Autodesk Inventor part; units mm, degrees
ref_plane "YZ Plane" through (0, 0, 0) normal (1, 0, 0) x (0, 1, 0)
ref_plane "XZ Plane" through (0, 0, 0) normal (0, 1, 0) x (-1, 0, 0)
ref_plane "XY Plane" through (0, 0, 0) normal (0, 0, 1) x (1, 0, 0)
sketch "Schizzo1" plane through (0, 0, 0) normal (0, 1, 0) x (-1, 0, 0)
  line L0 (-15, 6) -> (-15, 10.5)
  line L1 (-15, 10.5) -> (-11.5, 10.5)
  line L2 (-11.5, 10.5) -> (-11.5, 10)
  line L3 (-11.5, 10) -> (-10.2, 10)
  line L4 (-10.2, 10) -> (-10.2, 10.5)
  line L5 (-10.2, 10.5) -> (0, 10.5)
  line L6 (0, 10.5) -> (0, 6)
  line L7 (0, 6) -> (-15, 6)
  line L8 (0, 0) -> (5.7518, 0)
  dimension "d0" = 12
  dimension "d2" = 21
  dimension "d3" = 15
  dimension "d4" = 11.5
  dimension "d5" = 1.3
  dimension "d6" = 20
revolve "Rivoluzione1" add sketch "Schizzo1" angle 360 about axis through (0, 0, 0) along (-1, 0, 0)
fillet "Raccordo1" radius 0.2 1 edges at (15, 0, -10.5)
sketch "Schizzo2" plane through (15, 0, 0) normal (1, 0, 0) x (0, 0, -1)
  circle A0 centre (0, 0) radius 10.3
  circle A1 centre (0, 0) radius 9
  dimension "d13" = 18
extrude "Estrusione2" cut sketch "Schizzo2" against normal blind 1 contours A1
mirror "Specchio1" about plane through (0, 0, 8.25) normal (-1, 0, 0)
properties part number "LM10UU"
Work out the finished part from the listing and answer in its coordinate system (mm). A direction names the side the tool comes from. Coordinates: 2 decimals unless noted, no trailing zeros. Order: outer loops, then holes, each group sorted by start corner. A loop starts at its lowest first (then second) coordinate and runs counter-clockwise, first axis right, second up. Notation, with made-up numbers: M -18,67 L 20,67 A26 ccw 20,85 Z; hole C 70,-2 d11. An arc over 180 degrees is marked long. Use CSV: the item, a comma, the result in double quotes.
1) Section A-A on x = 6.5 is taken. Write down the section's boundary in (y, z), plus the area to 3 significant figures.
Worked out:
outline,"C 0,0 d21; hole C 0,0 d12"
area,"233 mm^2"
2) For faces 1 (the face through (-14, -6, 2)), 2 (the face through (10.84, -9.76, -2.17)), 3 (the face through (14.507, 8.923, 1.172)), 4 (the face through (-13.1, -3.2, 10)), determine the directions among +Z, -Z, +X, -X, +Y, -Y from which every point of the face is accessible in a straight line to the end or side of a thin tool.
Worked out:
face 1,"-X"
face 2,"none"
face 3,"+X"
face 4,"+X, -X"
3) Determine the mould class of faces 5 (the face through (13.1, 3.2, 10)), 6 (the face through (0, 0, -6)), 7 (the face through (-10.2, -9, -5)) for opening direction Y: released by +Y, released by -Y, zero draft, split by the parting line, or undercut.
Worked out:
face 5,"split by the parting line"
face 6,"undercut"
face 7,"zero draft"
4) Flat-ended cylindrical pins translate along their axes: pin 1 Ø3 at (y, z) = (5.5, 2.5) entering from +X; pin 2 Ø2 at (y, z) = (3, 7) entering from -X; pin 3 Ø1 at (x, y) = (2, -2) entering from -Z. Find the tip coordinate at first contact, or state that the pin passes through.
Worked out:
pin 1,"stops at x = 14"
pin 2,"stops at x = -14"
pin 3,"stops at z = -10.39"
5) Consider line 1 (X direction, y = -9.25, z = 4.75); line 2 (Y direction, x = -3, z = 0); line 3 (Y direction, x = -8.75, z = -3). Determine where each line is inside the solid, lowest interval first. Write a range as [from, to].
Worked out:
line 1,"x = [-14.97, -11.5], [-10.2, 10.2], [11.5, 14.97]"
line 2,"y = [-10.5, -6], [6, 10.5]"
line 3,"y = [-10.06, -5.2], [5.2, 10.06]"
